Autodesk Inventor part; units mm, degrees
ref_plane "YZ Plane" through (0, 0, 0) normal (1, 0, 0) x (0, 1, 0)
ref_plane "XZ Plane" through (0, 0, 0) normal (0, 1, 0) x (-1, 0, 0)
ref_plane "XY Plane" through (0, 0, 0) normal (0, 0, 1) x (1, 0, 0)
ref_plane "Work Plane1" through (0, 0, 0) normal (0, 0, 1) x (1, 0, 0)
sketch "Sketch1" plane through (0, 0, 0) normal (0, 0, 1) x (1, 0, 0)
  line L0 (-88.9, 0) -> (0, 0)
  line L1 (0, 0) -> (0, 38.1)
  line L2 (-88.9, 38.1) -> (0, 38.1)
  line L3 (-88.9, 0) -> (-88.9, 38.1)
  line L4 (0, 0) -> (2260.6, 0)
  line L5 (2260.6, 0) -> (2260.6, 38.1)
  line L6 (0, 38.1) -> (2260.6, 38.1)
  line L7 (0, 0) -> (0, 38.1)
  line L8 (2260.6, 0) -> (2349.5, 0)
  line L9 (2349.5, 0) -> (2349.5, 38.1)
  line L10 (2260.6, 38.1) -> (2349.5, 38.1)
  line L11 (2260.6, 0) -> (2260.6, 38.1)
  line L12 (1130.3, 38.1) -> (1130.3, 342.9)
  line L13 (1130.3, 342.9) -> (2349.5, 38.1)
  line L14 (1130.3, 342.9) -> (1121.0594, 305.9376)
  line L15 (1121.0594, 305.9376) -> (2192.4097, 38.1)
  point P0 (1130.3, 303.6274)
  dimension "d0" = 304.8
  dimension "d2" = 90
  dimension "d4" = 38.1
extrude "Extrusion1" add sketch "Sketch1" against normal blind 88.9 contours L6 L15 L12 L13 L10
properties part number "top head slant"
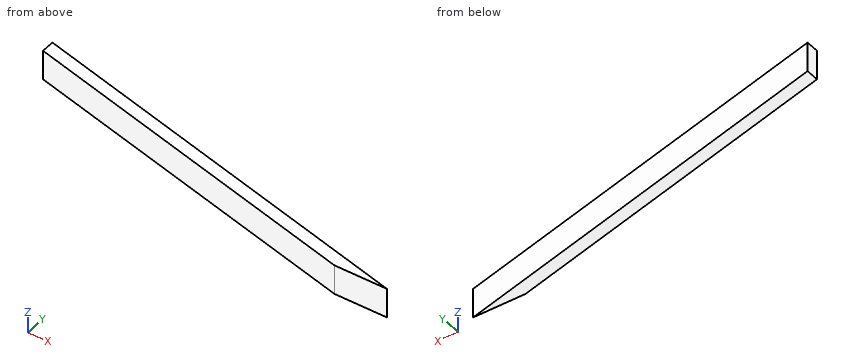
Model file for the job. Use its own axes, mm. Round coordinates to 2 decimals unless told otherwise and drop trailing zeros. Loops run counter-clockwise (first coordinate to the right, second up) from the corner with the lowest first, then second, coordinate; pieces in that order, holes last. Notation, with made-up numbers: M 44.5,-37.75 L 55.5,-37.75 A20 ccw 55.5,-18.75 Z; hole C 26,10 d3. An arc over 180 degrees is marked long. Put each result on its own line as item: value. Start each with the question number.
Item 1: Cut at B-B (y = 93). List the corners of the cut face in (x, z).
Item 2: Drill centre lines: line 1 along Y through (x, z) = (2125.5, -18.5); line 2 along Y through (x, z) = (1464.5, -24.5). Where is each one in solid material? Low to high.
Item 3: Cut at A-A (z = -54). List the corners of the cut face in (x, y).
Item 4: Drop flat-ended pins along their axis: P1, Ø3, axis at x = 1604, z = -65.5, coming from the -Y side; P2, Ø12, axis at x = 1533, z = -21.5, coming from the -Y side; P3, Ø8, axis at x = 1566, z = -14, coming from the +Y side (3 decimals). Give the stop position or say it passes through.
Answer block:
1. outline: M 1972.81,-88.9 L 2129.9,-88.9 L 2129.9,0 L 1972.81,0 Z
2. line 1: 54.83 to 94.1
2. line 2: 220.08 to 259.35
3. outline: M 1130.3,303.63 L 2192.41,38.1 L 2349.5,38.1 L 1130.3,342.9 Z
4. P1: y = 184.83
4. P2: y = 201.45
4. P3: y = 234.975
